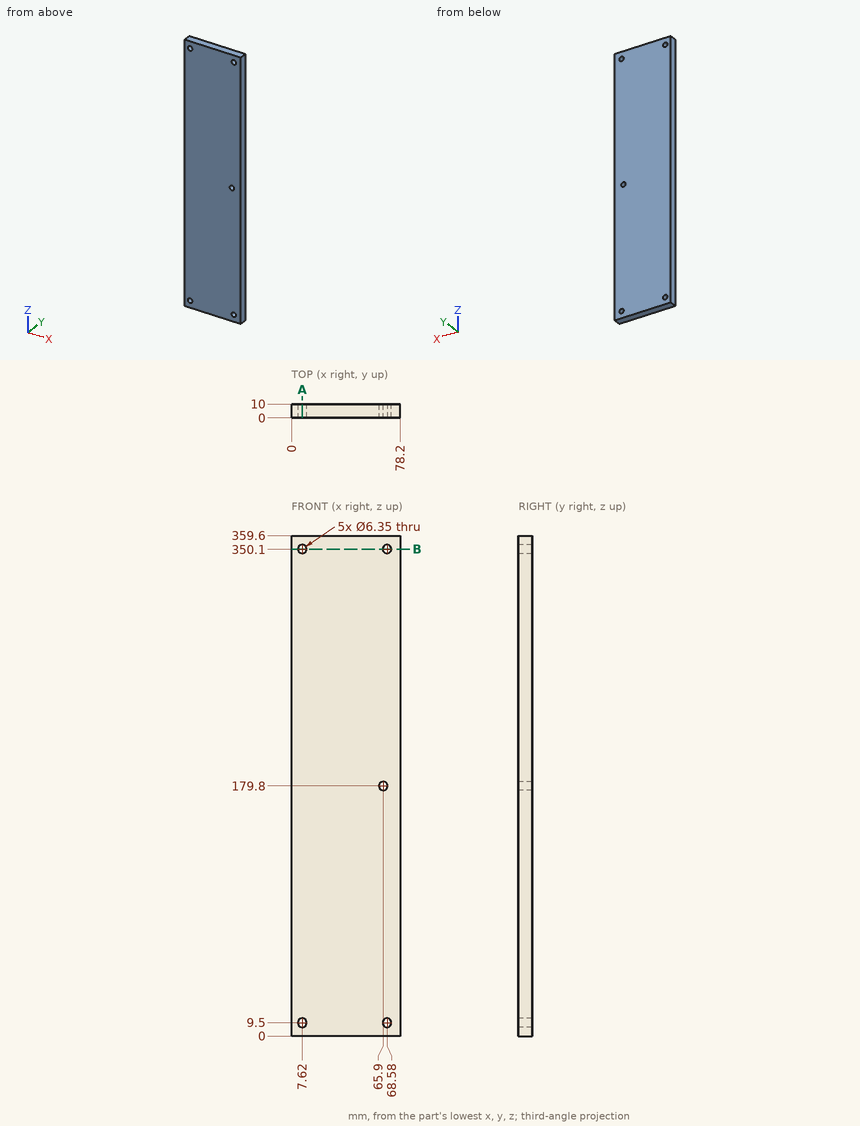
Here's the drawing with two shaded views (mm, measured from the low corner). I have some questions. Give positions to 0.01 mm unless a question says otherwise; leave off trailing zeros. Loops run counter-clockwise (first coordinate to the right, second up) from the corner with the lowest first, then second, coordinate; pieces in that order, holes last. Notation, with made-up numbers: (58, -7.5) - (63, -7.5) arc R19 cw to (63, 11.5) - close; hole circle Ø9 at (39, 24.5). An arc over 180 degrees is marked (long way). Answer in a Markdown table with one row per item. Add a question column.
Q1. If we section it at A-A (x = 7.62): List the corners of the cut face in (y, z) for me (3 decimals).
Q2. If we section it at B-B (z = 350.1): List the corners of the cut face in (x, y) for me (3 decimals).
Q3. Please list where these lines run through material, in increasing order: L1, parallel to X at y = 2, z = 350.1 (3 decimals); L2, parallel to Z at x = 7.62, y = 3.5 (3 decimals); L3, parallel to X at y = 4.5, z = 179.8 (3 decimals). Write a range as from..to.
The answers:
| question | item | result |
|---|---|---|
| 1 | outline | (0, 0) - (10, 0) - (10, 6.325) - (0, 6.325) - close; (0, 12.675) - (10, 12.675) - (10, 346.925) - (0, 346.925) - close; (0, 353.275) - (10, 353.275) - (10, 359.6) - (0, 359.6) - close |
| 2 | outline | (0, 0) - (4.445, 0) - (4.445, 10) - (0, 10) - close; (10.795, 0) - (65.405, 0) - (65.405, 10) - (10.795, 10) - close; (71.755, 0) - (78.2, 0) - (78.2, 10) - (71.755, 10) - close |
| 3 | L1 | x = 0..4.445, 10.795..65.405, 71.755..78.2 |
| 3 | L2 | z = 0..6.325, 12.675..346.925, 353.275..359.6 |
| 3 | L3 | x = 0..62.725, 69.075..78.2 |
